```python
from build123d import *

# Parameters (mm, degrees)
P_IDAT_VYSUNUT_M1_DEPTH   = 6
SKICA3_R                  = 8.5
SKICA3_R_2                = 2.425
ODEBRAT_VYSUNUT_M1_DEPTH  = 6
P_IDAT_VYSUNUT_M3_DEPTH   = 20
SKICA6_R                  = 14
ODEBRAT_VYSUNUT_M2_DEPTH  = 18.4
ODEBRAT_START             = -18.4
SKICA10_R                 = 14
ODEBRAT_VYSUNUT_M3_DEPTH  = 18.4
SKICA18_W                 = 15
SKICA18_H                 = 42
P_IDAT_VYSUNUT_M5_DEPTH   = 20
ODEBRAT_VYSUNUT_M9_DEPTH  = 20
SKICA14_R                 = 2.2
ODEBRAT_VYSUNUT_M7_DEPTH  = 5
ODEBRAT_START_2           = -5
SKICA15_R                 = 2.2
ODEBRAT_VYSUNUT_M8_DEPTH  = 5
SKICA23_R                 = 2.2
ODEBRAT_VYSUNUT_M10_DEPTH = 4
SKICA24_W                 = 18
SKICA24_H                 = 10.276194705
ODEBRAT_VYSUNUT_M12_DEPTH = 18.4
SKICA31_W                 = 22
SKICA31_H                 = 42
P_IDAT_VYSUNUT_M6_DEPTH   = 20
SKICA25_W                 = 18
SKICA25_H                 = 10.276194705
ODEBRAT_VYSUNUT_M13_DEPTH = 18.4
SKICA26_W                 = 20
SKICA26_H                 = 24
ODEBRAT_VYSUNUT_M14_DEPTH = 36.4
SKICA27_W                 = 20
SKICA27_H                 = 33
ODEBRAT_VYSUNUT_M15_DEPTH = 14


with BuildPart() as part:
    # Skica2 → Přidat vysunutím1 (new body)
    with BuildSketch(Plane.XY):
        with BuildLine():
            Line((2, 0), (129.6, 0))
            ThreePointArc((129.6, 0), (131.014213562, 0.585786438), (131.6, 2))
            Line((131.6, 2), (131.6, 84))
            ThreePointArc((131.6, 84), (131.014213562, 85.414213562), (129.6, 86))
            Line((129.6, 86), (2, 86))
            ThreePointArc((2, 86), (0.585786438, 85.414213562), (0, 84))
            Line((0, 84), (0, 2))
            ThreePointArc((0, 2), (0.585786438, 0.585786438), (2, 0))
        make_face()
    extrude(amount=P_IDAT_VYSUNUT_M1_DEPTH)

    # Skica3 → Odebrat vysunutím1 (cut)
    with BuildSketch(Plane.XY.offset(6)):
        with Locations((27, 43)):
            Circle(SKICA3_R)
        with Locations((127.6, 78.8)):
            Circle(SKICA3_R_2)
        with Locations((80, 7.2)):
            Circle(SKICA3_R_2)
        with Locations((127.6, 7.2)):
            Circle(SKICA3_R_2)
        with Locations((80, 78.8)):
            Circle(SKICA3_R_2)
    extrude(amount=-ODEBRAT_VYSUNUT_M1_DEPTH, mode=Mode.SUBTRACT)

    # Skica4 → Přidat vysunutím3 (add)
    with BuildSketch(Plane.XY.offset(6)):
        with BuildLine():
            Line((2, 86), (54, 86))
            Line((54, 86), (54, 64))
            Line((54, 64), (0, 64))
            Line((0, 64), (0, 84))
            ThreePointArc((0, 84), (0.585786438, 85.414213562), (2, 86))
        make_face()
        with BuildLine():
            Line((2, 0), (54, 0))
            Line((54, 0), (54, 22))
            Line((54, 22), (0, 22))
            Line((0, 22), (0, 2))
            ThreePointArc((0, 2), (0.585786438, 0.585786438), (2, 0))
        make_face()
    extrude(amount=P_IDAT_VYSUNUT_M3_DEPTH)

    # Skica6 → Odebrat vysunutím2 (cut)
    with BuildSketch(Plane.XZ):
        with Locations((27, 5)):
            Circle(SKICA6_R)
    extrude(amount=-ODEBRAT_VYSUNUT_M2_DEPTH, mode=Mode.SUBTRACT)

    # Skica10 → Odebrat vysunutím3 (cut)
    with BuildSketch(Plane(origin=(0, 86, 0), x_dir=(1, 0, 0), z_dir=(0, 1, 0)).offset(ODEBRAT_START)):
        with Locations((27, -5)):
            Circle(SKICA10_R)
    extrude(amount=ODEBRAT_VYSUNUT_M3_DEPTH, mode=Mode.SUBTRACT)

    # Skica18 → Přidat vysunutím5 (add)
    with BuildSketch(Plane.XY.offset(6)):
        with Locations((46.5, 43)):
            Rectangle(SKICA18_W, SKICA18_H)
    extrude(amount=P_IDAT_VYSUNUT_M5_DEPTH)

    # Skica21 → Odebrat vysunutím9 (cut)
    with BuildSketch(Plane.XY.offset(26)):
        with BuildLine():
            Line((39, 24), (39, 62))
            ThreePointArc((39, 62), (39.38, 61.620000112), (39.76, 62))
            ThreePointArc((39.76, 62), (40.36, 62.599999823), (40.96, 62))
            Line((40.96, 62), (40.96, 24))
            ThreePointArc((40.96, 24), (40.36, 23.4), (39.76, 24))
            ThreePointArc((39.76, 24), (39.38, 24.38), (39, 24))
        make_face()
    extrude(amount=-ODEBRAT_VYSUNUT_M9_DEPTH, mode=Mode.SUBTRACT)

    # Skica14 → Odebrat vysunutím7 (cut)
    with BuildSketch(Plane.XZ):
        with Locations(Location((9.3, 5, 0), (0, 0, 270))):
            Circle(SKICA14_R)
        with Locations(Location((44.7, 5, 0), (0, 0, 270))):
            Circle(SKICA14_R)
    extrude(amount=-ODEBRAT_VYSUNUT_M7_DEPTH, mode=Mode.SUBTRACT)

    # Skica15 → Odebrat vysunutím8 (cut)
    with BuildSketch(Plane(origin=(0, 86, 0), x_dir=(1, 0, 0), z_dir=(0, 1, 0)).offset(ODEBRAT_START_2)):
        with Locations(Location((9.3, -5, 0), (0, 0, 90))):
            Circle(SKICA15_R)
        with Locations(Location((44.7, -5, 0), (0, 0, 90))):
            Circle(SKICA15_R)
    extrude(amount=ODEBRAT_VYSUNUT_M8_DEPTH, mode=Mode.SUBTRACT)

    # Skica23 → Odebrat vysunutím10 (cut)
    with BuildSketch(Plane(origin=(0, 0, 0), x_dir=(-1, 0, 0), z_dir=(0, 0, -1))):
        with Locations((-118.8, 55.2)):
            Circle(SKICA23_R)
        with Locations((-88.8, 55.2)):
            Circle(SKICA23_R)
        with Locations((-88.8, 30.8)):
            Circle(SKICA23_R)
        with Locations((-118.8, 30.8)):
            Circle(SKICA23_R)
    extrude(amount=-ODEBRAT_VYSUNUT_M10_DEPTH, mode=Mode.SUBTRACT)

    # Skica24 → Odebrat vysunutím12 (cut)
    with BuildSketch(Plane(origin=(0, 86, 0), x_dir=(1, 0, 0), z_dir=(0, 1, 0))):
        with Locations((27, -20.861902648)):
            Rectangle(SKICA24_W, SKICA24_H)
    extrude(amount=-ODEBRAT_VYSUNUT_M12_DEPTH, mode=Mode.SUBTRACT)

    # Skica31 → Přidat vysunutím6 (add)
    with BuildSketch(Plane.XY.offset(6)):
        with Locations((65, 43)):
            Rectangle(SKICA31_W, SKICA31_H)
    extrude(amount=P_IDAT_VYSUNUT_M6_DEPTH)

    # Skica25 → Odebrat vysunutím13 (cut)
    with BuildSketch(Plane.XZ):
        with Locations((27, 20.861902648)):
            Rectangle(SKICA25_W, SKICA25_H)
    extrude(amount=-ODEBRAT_VYSUNUT_M13_DEPTH, mode=Mode.SUBTRACT)

    # Skica26 → Odebrat vysunutím14 (cut)
    with BuildSketch(Plane.ZY.offset(-40.96)):
        with Locations((16, 43)):
            Rectangle(SKICA26_W, SKICA26_H)
    extrude(amount=-ODEBRAT_VYSUNUT_M14_DEPTH, mode=Mode.SUBTRACT)

    # Skica27 → Odebrat vysunutím15 (cut)
    with BuildSketch(Plane.ZY.offset(-40.96)):
        with Locations((16, 43)):
            Rectangle(SKICA27_W, SKICA27_H)
    extrude(amount=-ODEBRAT_VYSUNUT_M15_DEPTH, mode=Mode.SUBTRACT)


solid = part.part
```
Geometry check sheet. Reference: the model listing, model coordinates, mm. A direction names the side the tool comes from. Give positions to 0.01 mm unless a question says otherwise; leave off trailing zeros. Loops run counter-clockwise (first coordinate to the right, second up) from the corner with the lowest first, then second, coordinate; pieces in that order, holes last. Notation, with made-up numbers: M -31.75,66.25 L -25.75,66.25 A23 ccw -25.75,105.25 Z; hole C 7,74.25 d6. An arc over 180 degrees is marked long. Answer as CSV lines item,"result".
Item 1: Depth check by flat-ended pin: P1, Ø2, axis at y = 61, z = 16.5, coming from the -X side; P2, Ø8, axis at x = 72, y = 15.5, coming from the +Z side; P3, Ø8, axis at x = 23, z = 9, coming from the -Y side. Enter the tip coordinate at first touch or a pass-through.
Values:
P1,"stops at x = 39"
P2,"stops at z = 6"
P3,"stops at y = 18.4"
Item 2: Cross-section at D-D on x = 9.3. Record the cut outline in (y, z), and give its area (3 significant figures).
Values:
outline,"M 0,0 L 86,0 L 86,2.8 L 81,2.8 L 81,7.2 L 86,7.2 L 86,26 L 64,26 L 64,6 L 22,6 L 22,26 L 0,26 L 0,7.2 L 5,7.2 L 5,2.8 L 0,2.8 Z"
area,"1,350 mm²"
Item 3: Cross-section at B-B on x = 27. Record the cut outline in (y, z).
Values:
outline,"M 18.4,0 L 34.5,0 L 34.5,6 L 22,6 L 22,26 L 18.4,26 Z; M 51.5,0 L 67.6,0 L 67.6,26 L 64,26 L 64,6 L 51.5,6 Z"
Item 4: Cross-section at C-C on y = 78.8. Record the cut outline in (x, z) (3 decimals), and give its area (3 significant figures).
Values:
outline,"M 0,0 L 13.923,0 A14 cw 18,15.724 L 18,26 L 0,26 Z; M 36,15.724 A14 cw 40.077,0 L 77.575,0 L 77.575,6 L 54,6 L 54,26 L 36,26 Z; M 82.425,0 L 125.175,0 L 125.175,6 L 82.425,6 Z; M 130.025,0 L 131.6,0 L 131.6,6 L 130.025,6 Z"
area,"1,220 mm²"
Item 5: Cross-section at A-A on y = 43. Record the cut outline in (x, z), and give its area (3 significant figures).
Values:
outline,"M 0,0 L 18.5,0 L 18.5,6 L 0,6 Z; M 35.5,0 L 131.6,0 L 131.6,6 L 35.5,6 Z"
area,"688 mm²"
Item 6: Access from +Z, -Z, +X, -X, +Y, -Y to the whole of each face (thin tool, end or side, straight path). Record for faces 5 (the flat face through (45, 81, 5)), 6 (the cylindrical face through (90.998, 55.297, 1.972)), 7 (the flat face through (65, 55, 16)), 8 (the cylindrical face through (40.58, 9.07, 8.4)).
Values:
face 5,"+Y"
face 6,"-Z"
face 7,"+Z, +X, -X"
face 8,"-Y"
Item 7: Release check for a two-part mould opening along Y. For faces 1 (the flat face through (27, 18.4, 10)), 2 (the flat face through (40.96, 61, 16)), 3 (the flat face through (0, 42, 4)), 4 (the flat face through (65, 31, 16)) record: pulls with the +Y half, pulls with the -Y half, needs draft (parallel to the pull), parting line crosses it, or undercut.
Values:
face 1,"pulls with the -Y half"
face 2,"undercut"
face 3,"needs draft"
face 4,"undercut"
Item 8: Material ranges on line 1 (X direction, y = 3.05, z = 5); line 2 (Y direction, x = 118.8, z = 0.95); line 3 (Z direction, x = 9, y = 1), recorded low to high.
Values:
line 1,"x = 0 to 7.1, 11.5 to 13, 41 to 42.5, 46.9 to 131.6"
line 2,"y = 0 to 28.6, 33 to 53, 57.4 to 86"
line 3,"z = 0 to 2.82, 7.18 to 26"
